For this review, take the finished solid that the model builds, in its own axes (mm). Round coordinates to 2 decimals unless told otherwise and drop trailing zeros. Order: outer loops, then holes, each group sorted by start corner. A loop starts at its lowest first (then second) coordinate and runs counter-clockwise, first axis right, second up. Notation, with made-up numbers: (19.25, -12) -> (76.25, -12) arc R16 ccw to (76.25, 12) -> close; hole circle Ø2 at (-8, 22). An arc over 180 degrees is marked (long way). Answer in a Markdown table with one row per item.
```python
from build123d import *

# Parameters (mm, degrees)
F1_DEPTH = 6


with BuildPart() as f1:
    # F0 (on Front) → F1 (new body)
    with BuildSketch(Plane.XZ):
        with BuildLine():
            Line((-250.833333, 48.124549), (-200, 0))
            Line((-200, 0), (200, 0))
            Line((200, 0), (250.833333, 48.124549))
            Line((250.833333, 48.124549), (330.833333, 48.124549))
            ThreePointArc((330.833333, 48.124549), (317.5363, 73.124549), (330.833333, 98.124549))
            Line((330.833333, 98.124549), (210.833333, 98.124549))
            Line((210.833333, 98.124549), (175, 50))
            Line((175, 50), (-175, 50))
            Line((-175, 50), (-210.833333, 98.124549))
            Line((-210.833333, 98.124549), (-330.833333, 98.124549))
            ThreePointArc((-330.833333, 98.124549), (-321.067327, 87.282684), (-317.5363, 73.124549))
            ThreePointArc((-317.5363, 73.124549), (-321.067327, 58.966415), (-330.833333, 48.124549))
            Line((-330.833333, 48.124549), (-250.833333, 48.124549))
        make_face()
    extrude(amount=F1_DEPTH)


solid = f1.part
```
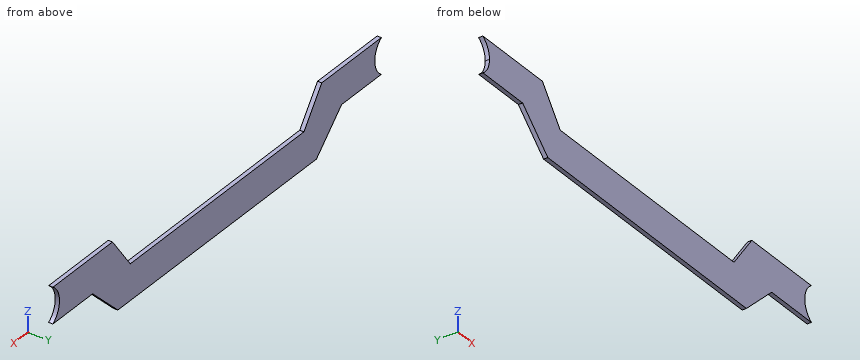
Q1. To check wall thickness, follow probe 1 along Z at (x, y) = (27, -1.9); probe 2 along X at (y, z) = (-3.3, 91.5); probe 3 along Z at (x, y) = (273, -0.75). State the ranges of each line that lie inside material, in increasing order.
Answer key:
| item | result |
|---|---|
| probe 1 | z = 0 to 50 |
| probe 2 | x = -323.78 to -205.9, 205.9 to 323.78 |
| probe 3 | z = 48.12 to 98.12 |
Q2. Take a section at D-D, the plane z = 39.5. Write out the cut boundary in (x, y).
Answer key:
| item | result |
|---|---|
| outline | (-241.72, -6) -> (241.72, -6) -> (241.72, 0) -> (-241.72, 0) -> close |
Q3. Clearance check with flat-ended pins moving along their axes: pin 1 Ø3 at (y, z) = (-1.5, 65) entering from +X; pin 2 Ø1.8 at (x, y) = (293, -4.5) entering from -Z. State where each tip first meets the part, or that it passes through.
Answer key:
| item | result |
|---|---|
| pin 1 | stops at x = 319.11 |
| pin 2 | stops at z = 48.12 |
Q4. Take a section at A-A, the plane z = 91. Write out the cut boundary in (x, y), then the cut area to 3 significant figures.
Answer key:
| item | result |
|---|---|
| outline | (-323.41, -6) -> (-205.53, -6) -> (-205.53, 0) -> (-323.41, 0) -> close; (205.53, -6) -> (323.41, -6) -> (323.41, 0) -> (205.53, 0) -> close |
| area | 1,410 mm^2 |
Q5. Take a section at B-B, the plane y = -3. Write out the cut boundary in (x, z), then the cut area to 3 significant figures.
Answer key:
| item | result |
|---|---|
| outline | (-330.83, 48.12) -> (-250.83, 48.12) -> (-200, 0) -> (200, 0) -> (250.83, 48.12) -> (330.83, 48.12) arc R30.15 cw to (330.83, 98.12) -> (210.83, 98.12) -> (175, 50) -> (-175, 50) -> (-210.83, 98.12) -> (-330.83, 98.12) arc R30.15 cw to (-317.54, 73.12) arc R30.15 cw to start |
| area | 35,300 mm^2 |
Q6. Take a section at C-C, the plane x = 31.5. Write out the cut boundary in (y, z), then the cut area to 3 significant figures.
Answer key:
| item | result |
|---|---|
| outline | (-6, 0) -> (0, 0) -> (0, 50) -> (-6, 50) -> close |
| area | 300 mm^2 |
